Work out the finished part from the listing and answer in its coordinate system (mm). Face numbers are marked on the shaded views. A direction names the side the tool comes from. Round coordinates to 2 decimals unless told otherwise and drop trailing zeros. Loops run counter-clockwise (first coordinate to the right, second up) from the corner with the lowest first, then second, coordinate; pieces in that order, holes last. Notation, with made-up numbers: (-32, -13.5) - (-24, -13.5) arc R11 cw to (-24, -6.5) - close; hole circle Ø3 at (-13.75, -0.75). An arc over 180 degrees is marked (long way). Return JSON: item names as keys, results as strings.
from build123d import *

# Parameters (mm, degrees)
BOSS_EXTRUDE1_DEPTH = 119.38
CUT_EXTRUDE1_DEPTH  = 115.57
SKETCH5_W           = 84.328
SKETCH5_H           = 105.41
CUT_EXTRUDE4_DEPTH  = 19.05
CUT_EXTRUDE5_START  = -24.13
CUT_EXTRUDE5_DEPTH  = 43.18
CUT_EXTRUDE6_DEPTH  = 43.18
FILLET2_R           = 2.54
FILLET3_R           = 1.27


with BuildPart() as part:
    # Sketch1 → Boss-Extrude1 (new body)
    with BuildSketch(Plane(origin=(0, 0, 0), x_dir=(1, 0, 0), z_dir=(0, 1, 0))):
        Polygon((0, 64.516), (13.97, 70.866), (13.97, 43.434), (0, 49.784), (0, 0), (127, 0), (127, 114.3), (0, 114.3), align=None)
    extrude(amount=BOSS_EXTRUDE1_DEPTH)

    # Sketch2 → Cut-Extrude1 (cut)
    with BuildSketch(Plane(origin=(0, 119.38, 0), x_dir=(1, 0, 0), z_dir=(0, 1, 0))):
        with BuildLine():
            Line((20.32, 77.47), (104.648, 77.47))
            Line((104.648, 77.47), (104.648, 67.31))
            ThreePointArc((104.648, 67.31), (123.698, 48.26), (104.648, 29.21))
            Line((104.648, 29.21), (104.648, 19.05))
            Line((104.648, 19.05), (20.32, 19.05))
            Line((20.32, 19.05), (20.32, 77.47))
        make_face()
    extrude(amount=-CUT_EXTRUDE1_DEPTH, mode=Mode.SUBTRACT)

    # Sketch5 → Cut-Extrude4 (cut)
    with BuildSketch(Plane(origin=(0, 119.38, 0), x_dir=(1, 0, 0), z_dir=(0, 1, 0))):
        with Locations((62.484, 57.15)):
            Rectangle(SKETCH5_W, SKETCH5_H)
    extrude(amount=-CUT_EXTRUDE4_DEPTH, mode=Mode.SUBTRACT)

    # Sketch6 → Cut-Extrude5 (cut)
    with BuildSketch(Plane(origin=(0, 100.33, 0), x_dir=(1, 0, 0), z_dir=(0, 1, 0)).offset(CUT_EXTRUDE5_START)):
        with BuildLine():
            Line((6.35, 106.68), (114.3, 106.68))
            Line((114.3, 106.68), (114.3, 102.87))
            ThreePointArc((114.3, 102.87), (123.823120388, 93.346879612), (114.3, 83.823759224))
            Line((114.3, 83.823759224), (114.3, 80.01))
            Line((114.3, 80.01), (6.35, 80.01))
            Line((6.35, 80.01), (6.35, 106.68))
        make_face()
    extrude(amount=CUT_EXTRUDE5_DEPTH, mode=Mode.SUBTRACT)

    # Sketch6<2> → Cut-Extrude6 (cut)
    with BuildSketch(Plane(origin=(0, 100.33, 0), x_dir=(1, 0, 0), z_dir=(0, 1, 0))):
        with BuildLine():
            Line((6.35, 106.68), (114.3, 106.68))
            Line((114.3, 106.68), (114.3, 102.87))
            ThreePointArc((114.3, 102.87), (123.823120388, 93.346879612), (114.3, 83.823759224))
            Line((114.3, 83.823759224), (114.3, 80.01))
            Line((114.3, 80.01), (6.35, 80.01))
            Line((6.35, 80.01), (6.35, 106.68))
        make_face()
    extrude(amount=-CUT_EXTRUDE6_DEPTH, mode=Mode.SUBTRACT)

    # Fillet2
    fillet2_edges = [part.edges().sort_by_distance(p)[0] for p in [
        (127, 119.38, -57.15),
        (127, 59.69, -114.3),
        (127, 59.69, 0),
        (63.5, 119.38, -114.3),
        (63.5, 119.38, 0),
    ]]
    fillet(fillet2_edges, radius=FILLET2_R)

    # Fillet3
    fillet3_edges = [part.edges().sort_by_distance(p)[0] for p in [
        (20.32, 52.07, -19.05),
        (20.32, 52.07, -77.47),
        (104.648, 61.595, -67.31),
        (104.648, 61.595, -29.21),
        (104.648, 52.07, -19.05),
        (20.32, 109.855, -4.445),
        (104.648, 109.855, -109.855),
        (20.32, 109.855, -109.855),
        (104.648, 109.855, -4.445),
        (104.648, 109.855, -106.68),
        (6.35, 88.265, -106.68),
        (20.32, 109.855, -106.68),
        (114.3, 88.265, -106.68),
        (114.3, 88.265, -102.87),
        (114.3, 88.265, -83.823759224),
        (114.3, 88.265, -80.01),
    ]]
    fillet(fillet3_edges, radius=FILLET3_R)


solid = part.part
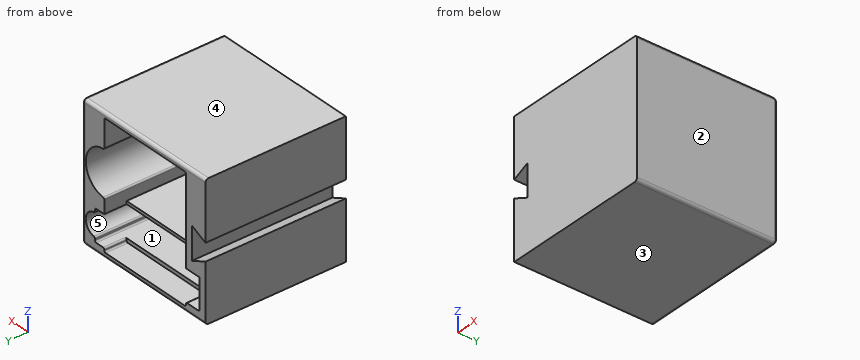
1) A tool of negligible diameter and unlimited length cuts with its end or side. For the marked faces 1 and 2, from which of +Z, -Z, +X, -X, +Y, -Y can it reach the whole face along a straight path? Write none if from no direction.
Verdict:
{"face 1": "+Y", "face 2": "+Z, -Z, +X, +Y, -Y"}
2) Find the intervals of material crossed by L1, parallel to Z at x = 83, y = 14; L2, parallel to Z at x = 19.5, y = 60; L3, parallel to Z at x = 110, y = 89, in increasing order.
Verdict:
{"L1": "z = -114.3 to -77.47, -19.05 to 0", "L2": "z = -114.3 to -106.68, -80.01 to 0", "L3": "z = -114.3 to -106.68, -80.01 to -66.54, -29.98 to 0"}
3) Section D-D (z = -48) is taken. Give the vertices of the cut face in (x, y), and give its area (3 significant figures).
Verdict:
{"outline": "(0, 0) - (3.92, 0) - (3.92, 119.38) - (0, 119.38) - close; (13.97, 0) - (127, 0) - (127, 116.84) arc R2.54 ccw to (124.46, 119.38) - (123.7, 119.38) - (123.7, 3.81) - (20.32, 3.81) - (20.32, 119.38) - (13.97, 119.38) - close", "area": "2,010 mm2"}
4) Section C-C (x = 31) is taken. Give the vertices of the cut face in (y, z) (3 decimals), and give its area (3 significant figures).
Verdict:
{"outline": "(0, -114.3) - (116.84, -114.3) arc R2.54 ccw to (119.38, -111.76) - (119.38, -109.855) - (100.33, -109.855) - (100.33, -106.68) - (57.15, -106.68) - (57.15, -80.01) - (100.33, -80.01) - (100.33, -77.47) - (3.81, -77.47) - (3.81, -19.05) - (100.33, -19.05) - (100.33, -4.445) - (119.38, -4.445) - (119.38, -2.54) arc R2.54 ccw to (116.84, 0) - (0, 0) - close", "area": "4,840 mm2"}
5) Flat-ended cylindrical pins translate along their axes: pin 1 (1 mm diameter, centred on y = 22.5, z = -46, fed in from -X); pin 2 (1.1 mm diameter, centred on x = 67.5, z = -78.5, fed in from +Y); pin 3 (13.5 mm diameter, centred on x = 57.5, z = -94.5, fed in from +Y); pin 4 (5 mm diameter, centred on x = 100.5, z = -23.5, fed in from +Y). Find the tip coordinate at first contact, or state that the pin passes through.
Verdict:
{"pin 1": "stops at x = 0", "pin 2": "stops at y = 100.33", "pin 3": "stops at y = 57.15", "pin 4": "stops at y = 3.81"}
6) Determine the mould class of the marked faces 3, 4 and 5 for opening direction Z: pulls with the +Z half, pulls with the -Z half, needs draft (parallel to the pull), parting line crosses it, or undercut.
Verdict:
{"face 3": "pulls with the -Z half", "face 4": "pulls with the +Z half", "face 5": "undercut"}
7) Section A-A (y = 35.5) is taken. Give the vertices of the cut face in (x, z).
Verdict:
{"outline": "(0, -114.3) - (124.46, -114.3) arc R2.54 ccw to (127, -111.76) - (127, -2.54) arc R2.54 ccw to (124.46, 0) - (0, 0) - (0, -49.78) - (13.97, -43.43) - (13.97, -70.87) - (0, -64.52) - close; hole (20.32, -76.2) arc R1.27 ccw to (21.59, -77.47) - (104.65, -77.47) - (104.65, -68.54) arc R1.27 cw to (105.84, -67.27) arc R19.05 ccw to (105.84, -29.25) arc R1.27 cw to (104.65, -27.98) - (104.65, -20.32) arc R1.27 ccw to (103.38, -19.05) - (21.59, -19.05) arc R1.27 ccw to (20.32, -20.32) - close"}
8) Section B-B (y = 81.5) is taken. Count the separate pieces of the cut face and the enclosed holes in it, and give its area (3 significant figures).
Verdict:
{"separate pieces": "1", "enclosed holes": "2", "area": "5,700 mm2"}
